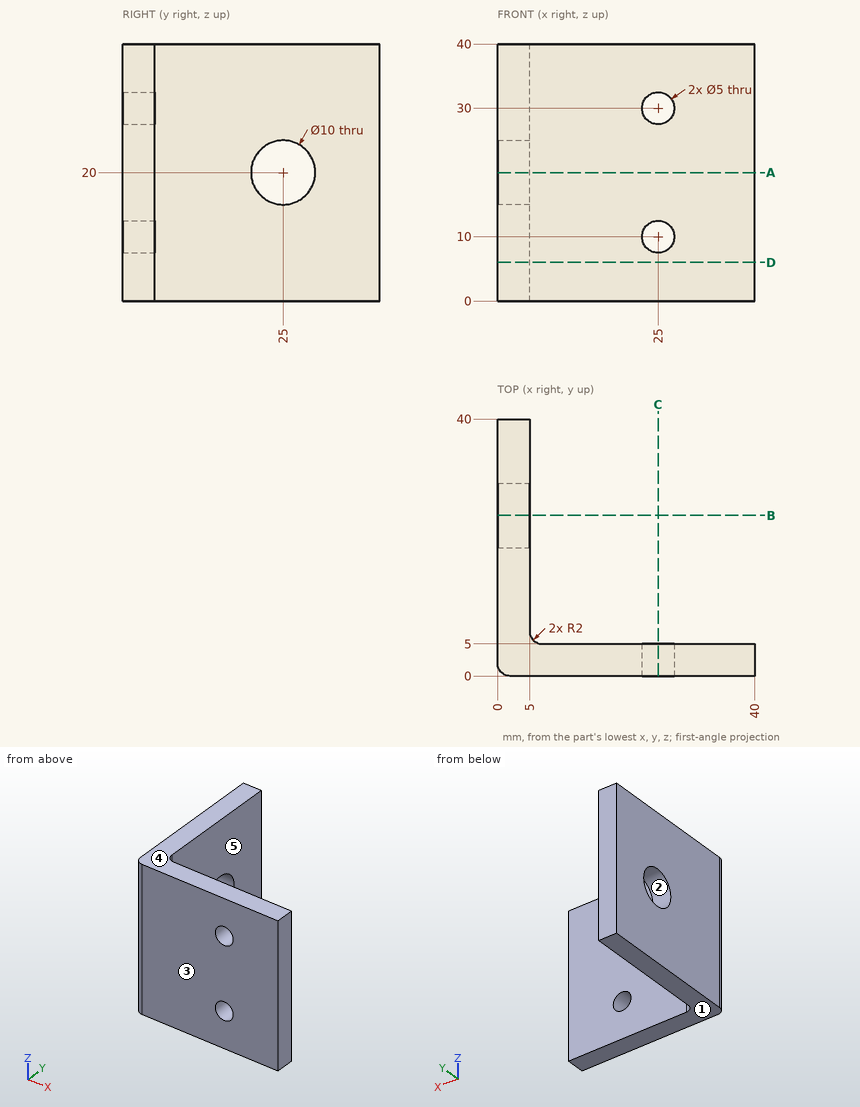
Check sheet for the drawn part. Datum: minimum x, y, z corner. Units: mm. A direction names the side the tool comes from. Round coordinates to 2 decimals unless told otherwise and drop trailing zeros. Loops run counter-clockwise (first coordinate to the right, second up) from the corner with the lowest first, then second, coordinate; pieces in that order, holes last. Notation, with made-up numbers: M -37,21 L -31,21 A18 ccw -31,55 Z; hole C 57.5,46 d6. An arc over 180 degrees is marked long. Write each question's results on one line, items separated by ' | '.
1) Mould release check, pull along Z, two halves, no side actions. Record for the marked faces 1, 2 and 3: released by +Z, released by -Z, zero draft, split by the parting line, or undercut.
Checks:
face 1: released by -Z | face 2: undercut | face 3: zero draft
2) Section check A-A on z = 20. Record the boundary of the cut face in (x, y).
Checks:
outline: M 0,2 A2 ccw 2,0 L 40,0 L 40,5 L 7,5 A2 cw 5,7 L 5,20 L 0,20 Z; M 0,30 L 5,30 L 5,40 L 0,40 Z
3) Access from +Z, -Z, +X, -X, +Y, -Y to the whole of each face (thin tool, end or side, straight path). Record for the marked faces 4 and 5.
Checks:
face 4: +Z, +X, -X, +Y, -Y | face 5: +Z, -Z, +X, +Y
4) Section check B-B on y = 25. Record the boundary of the cut face in (x, z), then the cut area to 3 significant figures.
Checks:
outline: M 0,0 L 5,0 L 5,15 L 0,15 Z; M 0,25 L 5,25 L 5,40 L 0,40 Z | area: 150 mm2
5) Section check D-D on z = 6. Record the boundary of the cut face in (x, y).
Checks:
outline: M 0,2 A2 ccw 2,0 L 40,0 L 40,5 L 7,5 A2 cw 5,7 L 5,40 L 0,40 Z
6) Section check C-C on x = 25. Record the boundary of the cut face in (y, z), then the cut area to 3 significant figures.
Checks:
outline: M 0,0 L 5,0 L 5,7.5 L 0,7.5 Z; M 0,12.5 L 5,12.5 L 5,27.5 L 0,27.5 Z; M 0,32.5 L 5,32.5 L 5,40 L 0,40 Z | area: 150 mm2
7) Scan lines: L1, parallel to Z at x = 25, y = 2.4; L2, parallel to X at y = 2, z = 10; L3, parallel to Y at x = 2, z = 20. Record each from-to range of solid material in increasing order. Write a range as from..to.
Checks:
L1: z = 0..7.5, 12.5..27.5, 32.5..40 | L2: x = 0..22.5, 27.5..40 | L3: y = 0..20, 30..40
8) Gauge pin test, flat ends, axial feed: P1, Ø8, axis at x = 25, z = 30, coming from the -Y side; P2, Ø8, axis at x = 25, z = 10, coming from the +Y side; P3, Ø10, axis at y = 31.5, z = 20, coming from the +X side; P4, Ø6, axis at y = 25, z = 20, coming from the -X side. Record the tip position at first contact, or that the pin passes through.
Checks:
P1: stops at y = 0 | P2: stops at y = 5 | P3: stops at x = 5 | P4: passes through
